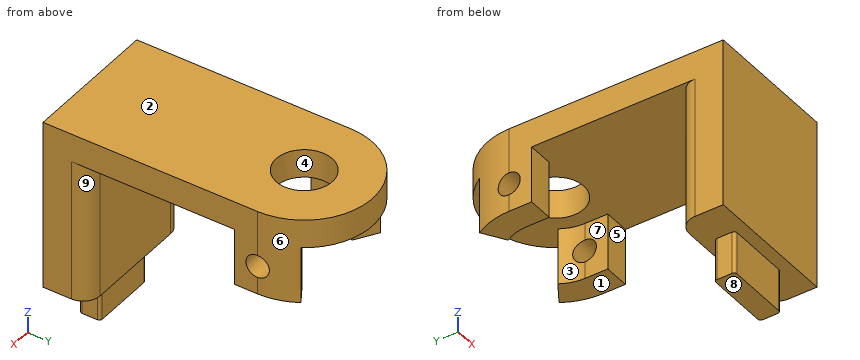
Autodesk Inventor part; units mm, degrees
ref_plane "YZ Plane" through (0, 0, 0) normal (1, 0, 0) x (0, 1, 0)
ref_plane "XZ Plane" through (0, 0, 0) normal (0, 1, 0) x (-1, 0, 0)
ref_plane "XY Plane" through (0, 0, 0) normal (0, 0, 1) x (1, 0, 0)
sketch "Sketch1" plane through (0, 0, 0) normal (0, 0, 1) x (1, 0, 0)
  line L0 (-12, 0) -> (12, 0)
  line L1 (12, 0) -> (12, 37.7)
  arc A0 (12, 37.7) -> (-12, 37.7) centre (0, 37.7) ccw
  line L2 (-12, 37.7) -> (-12, 0)
  circle A1 centre (0, 37.7) radius 4.925
  line L3 (12, 8) -> (-12, 8)
  line L4 (6, 6) -> (-6, 6) construction
  line L5 (-6, 6) -> (-6, 2) construction
  line L6 (-6, 2) -> (6, 2) construction
  line L7 (6, 2) -> (6, 6) construction
  line L8 (-5.84, 2.16) -> (-5.84, 5.84)
  line L9 (-5.84, 5.84) -> (5.84, 5.84)
  line L10 (5.84, 5.84) -> (5.84, 2.16)
  line L11 (5.84, 2.16) -> (-5.84, 2.16)
  point P0 (0, 0)
  point P1 (0, 0)
  point P2 (0, 2)
  dimension "d0" = 24
  dimension "d1" = 37.7
  dimension "d2" = 9.85
  dimension "d5" = 8
  dimension "d6" = 2
  dimension "d7" = 4
  dimension "d8" = 12
  dimension "d9" = 0.16
extrude "Extrusion1" add sketch "Sketch1" along normal blind 5 contours L2 L3 L1 L0 | L2 A0 L1 L3 | L8 L9 L10 L11
extrude "Extrusion2" add sketch "Sketch1" against normal blind 25 contours L2 L3 L1 L0 | L8 L9 L10 L11
sketch "Sketch3" plane through (0, 0, -25) normal (0, 0, -1) x (-1, 0, 0)
  line L0 (-5.84, 5.84) -> (-5.84, 2.16)
  line L1 (5.84, 5.84) -> (-5.84, 5.84)
  line L2 (5.84, 2.16) -> (5.84, 5.84)
  line L3 (-5.84, 2.16) -> (5.84, 2.16)
  point P0 (0, 0)
extrude "Extrusion3" add sketch "Sketch3" along normal blind 7.5
fillet "Fillet1" radius 0.5 4 edges at (-5.84, 5.84, -28.75) (-5.84, 2.16, -28.75) (5.84, 2.16, -28.75) (5.84, 5.84, -28.75)
fillet "Fillet2" radius 3 2 edges at (-12, 8, -12.5) (12, 8, -12.5)
sketch "Sketch4" plane through (0, 0, 0) normal (0, 0, -1) x (-1, 0, 0)
  line L0 (0, 41.7) -> (17.7659, 41.7) construction
  line L1 (17.7659, 41.7) -> (17.7659, 33.7) construction
  line L2 (17.7659, 33.7) -> (12, 33.7) construction
  line L3 (0, 33.7) -> (0, 41.7) construction
  arc A0 (12, 37.7) -> (-12, 37.7) centre (0, 37.7) ccw
  line L4 (12, 37.7) -> (12, 0)
  arc A1 (7.5, 37.7) -> (6.3443, 41.7) centre (0, 37.7) ccw
  line L5 (7.5, 37.7) -> (7.5, 33.7)
  line L6 (6.3443, 41.7) -> (10.1509, 44.1)
  line L7 (7.5, 33.7) -> (0, 33.7) construction
  line L8 (12, 33.7) -> (7.5, 33.7)
  arc A2 (6.3443, 41.7) -> (-7.5, 37.7) centre (0, 37.7) ccw construction
  line L9 (7.5, 33.7) -> (7.5, 0) construction
  point P0 (0, 0)
  point P1 (17.7659, 37.7)
  dimension "d16" = 8
  dimension "d17" = 4.5
extrude "Extrusion4" add sketch "Sketch4" along normal blind 10
mirror "Mirror1" about plane through (0, 0, 0) normal (1, 0, 0) of "Extrusion4"
sketch "Sketch5" plane through (0, 0, 0) normal (1, 0, 0) x (0, 1, 0)
  line L0 (32.775, 5) -> (42.625, 5)
  line L1 (42.625, 0) -> (32.775, 0)
  circle A0 centre (37.7, -5) radius 2
  line L2 (41.7, 0) -> (41.7, -10)
  point P0 (0, 0)
  point P1 (41.7, -5)
  point P2 (37.7, 5)
  dimension "d20" = 4
extrude "Extrusion5" cut sketch "Sketch5" along normal through all both and the other way through all
properties part number "Casing Attachment MH" material "Aluminum 6061"
Verification items for the finished model (mm, model axes). Face numbers are marked on the shaded views. A direction names the side the tool comes from. Give positions to 0.01 mm unless a question says otherwise; leave off trailing zeros. Loops run counter-clockwise (first coordinate to the right, second up) from the corner with the lowest first, then second, coordinate; pieces in that order, holes last. Notation, with made-up numbers: (70.25, 85) - (91.25, 85) arc R21 ccw to (91.25, 117) - close; hole circle Ø8 at (-23.75, 26.5). An arc over 180 degrees is marked (long way). Write item = value, one per line. Start each with the question number.
Q1. Depth check by flat-ended pin: P1, Ø8, axis at x = -6.5, y = 41, coming from the -Z side; P2, Ø6, axis at x = 0.5, z = -27, coming from the +Y side; P3, Ø1, axis at x = -5, z = -28, coming from the +Y side. Enter the tip coordinate at first touch or a pass-through.
Q2. Cross-section at D-D, the plane y = 20. Enter the section's corners in (x, z), and give its area (3 significant figures).
Q3. Mould release check, pull along X, two halves, no side actions. Record for the marked faces 6, 7, 8 and 9: released by +X, released by -X, zero draft, split by the parting line, or undercut.
Q4. Thickness scan on line 1 (Z direction, x = -8.3, y = 37.7); line 2 (Y direction, x = 9.8, z = -5); line 3 (Y direction, x = -2, z = -12). Record the ranges inside material, lowest first.
Q5. Tool access check on the marked faces 1, 2, 3, 4 and 5. Record the directions out of +Z, -Z, +X, -X, +Y, -Y that give a thin tool (end or side, any length) a straight path to the whole face; none if there is none.
Q6. Cross-section at C-C, the plane z = -22. Enter the section's corners in (x, y), and give its area (3 significant figures).
Q7. Cross-section at B-B, the plane z = -2. Enter the section's corners in (x, y), and give its area (4 significant figures).
Q8. Cross-section at A-A, the plane x = 0. Enter the section's corners in (y, z) (3 decimals), and give its area (3 significant figures).
Answer key:
q1.P1 = -10
q1.P2 = 8
q1.P3 = 5.84
q2.outline = (-12, 0) - (12, 0) - (12, 5) - (-12, 5) - close
q2.area = 120 mm^2
q3.face_6 = split by the parting line
q3.face_7 = undercut
q3.face_8 = zero draft
q3.face_9 = released by +X
q4.line_1 = -10 to -7, -3 to 5
q4.line_2 = 0 to 7.89, 33.7 to 35.7, 39.7 to 43.88
q4.line_3 = 0 to 8
q5.face_1 = -Z, +X, -X, +Y
q5.face_2 = +Z, +X, -X, +Y, -Y
q5.face_3 = -Z
q5.face_4 = +Z, -Z
q5.face_5 = -Z, +X, -X
q6.outline = (-12, 0) - (12, 0) - (12, 5) arc R3 ccw to (9, 8) - (-9, 8) arc R3 ccw to (-12, 5) - close
q6.area = 188 mm^2
q7.outline = (-12, 0) - (12, 0) - (12, 5) arc R3 ccw to (9, 8) - (-9, 8) arc R3 ccw to (-12, 5) - close; (-12, 33.7) - (-7.5, 33.7) - (-7.5, 37.7) arc R7.5 cw to (-6.34, 41.7) - (-10.15, 44.1) arc R12 ccw to (-12, 37.7) - close; (6.34, 41.7) arc R7.5 cw to (7.5, 37.7) - (7.5, 33.7) - (12, 33.7) - (12, 37.7) arc R12 ccw to (10.15, 44.1) - close
q7.area = 273.5 mm^2
q8.outline = (0, -25) - (2.16, -25) - (2.16, -32.5) - (5.84, -32.5) - (5.84, -25) - (8, -25) - (8, 0) - (32.775, 0) - (32.775, 5) - (0, 5) - close; (42.625, 0) - (49.7, 0) - (49.7, 5) - (42.625, 5) - close
q8.area = 427 mm^2
